Autodesk Inventor part; units mm, degrees
ref_plane "YZ Plane" through (0, 0, 0) normal (1, 0, 0) x (0, 1, 0)
ref_plane "XZ Plane" through (0, 0, 0) normal (0, 1, 0) x (-1, 0, 0)
ref_plane "XY Plane" through (0, 0, 0) normal (0, 0, 1) x (1, 0, 0)
sketch "Sketch1" plane through (0, 0, 0) normal (0, 0, 1) x (1, 0, 0)
  line L0 (-50, -57.5) -> (50, -57.5)
  line L1 (50, -57.5) -> (50, 57.5)
  line L2 (50, 57.5) -> (-50, 57.5)
  line L3 (-50, 57.5) -> (-50, -57.5)
  line L4 (-50, -57.5) -> (50, 57.5) construction
  line L5 (50, -57.5) -> (-50, 57.5) construction
  point P0 (0, 0)
  dimension "d0" = 100
  dimension "d1" = 115
extrude "Plate1" add sketch "Sketch1" along normal blind 3
sketch "Sketch5" plane through (0, 0, 3) normal (0, 0, 1) x (1, 0, 0)
  line L0 (50, -57.5) -> (-50, -57.5) construction
  line L1 (50, 57.5) -> (50, -57.5) construction
  line L2 (-50, 57.5) -> (50, 57.5) construction
  line L3 (-50, -57.5) -> (-50, 57.5) construction
  line L4 (50, 57.5) -> (-50, 57.5) construction
  line L5 (-50, 57.5) -> (50, -57.5) construction
  line L6 (-39.5011, 45.4263) -> (-32.9394, 37.8803) construction
  line L7 (-44.0288, 41.4892) -> (-37.467, 33.9432)
  line L8 (-28.4117, 41.8173) -> (-34.9735, 49.3634)
  arc A0 (-34.9735, 49.3634) -> (-44.0288, 41.4892) centre (-39.5011, 45.4263) ccw
  arc A1 (-37.467, 33.9432) -> (-28.4117, 41.8173) centre (-32.9394, 37.8803) ccw
  point P0 (0, 0)
  point P1 (-36.2202, 41.6533)
  dimension "d22" = 12
  dimension "d23" = 10
  dimension "d24" = 16
extrude "Cut1" cut sketch "Sketch5" against normal blind 3
mirror "Mirror1" about plane through (0, 0, 0) normal (0, 1, 0) of "Cut1"
mirror "Mirror2" about plane through (0, 0, 0) normal (1, 0, 0) of "Cut1", "Mirror1"
fillet "Corner Round1" radius 8 4 edges at (-50, 57.5, 1.5) (50, 57.5, 1.5) (50, -57.5, 1.5) (-50, -57.5, 1.5)
equation "\"d25\" = Thickness"
equation "\"d2\" = Thickness"
equation "\"BendReliefWidth\" = Thickness"
equation "\"BendReliefDepth\" = 0.5 * Thickness"
equation "\"CornerReliefSize\" = 4 * Thickness"
equation "\"MinimumRemnant\" = 2 * Thickness"
equation "\"TransitionRadius\" = BendRadius"
equation "\"JacobiRadiusSize\" = BendRadius"
equation "\"GapSize\" = Thickness"
properties part number "AQUA AISI304 4vv wheel plate 150" material "Stainless Steel"
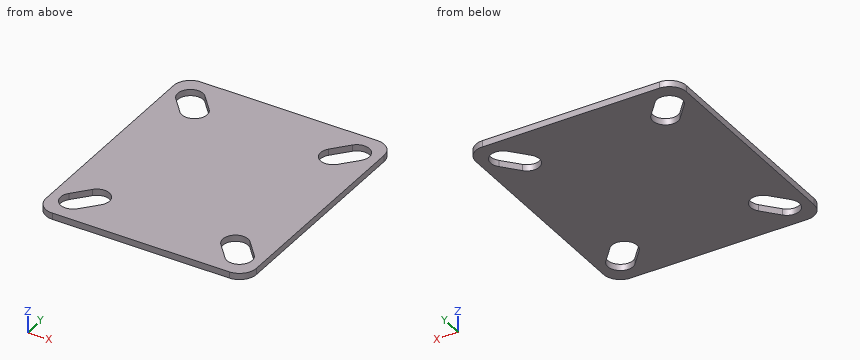
Here's how the part is built. I have some questions about the finished solid (model axes, mm). Coordinates: 2 decimals unless noted, no trailing zeros. Write each loop counter-clockwise with the first axis right and the second up, starting at its lowest first coordinate (ties: lowest second). Pieces come first, ordered by that corner, then holes.
Item 1: I want a section at A-A on z = 1.05. Write out the boundary of the cut face in (x, y).
Item 2: Will this pin go through, and if not, where does the flat tip stop? pin 1 (5 mm diameter, centred on x = 9, y = 16, fed in from -Z).
Item 3: I want a section at C-C on x = -30.5. Write out the boundary of the cut face in (y, z).
Item 4: I want a section at B-B on x = 30. Write out the boundary of the cut face in (y, z), and give its area (3 significant figures).
Item 5: If I drill on line 1 (X direction, y = -39, z = 1.7); line 2 (Y direction, x = 39, z = 0.8); line 3 (Y direction, x = -38, z = 0.95), over which ranges is the centre line in solid material (lowest first)?
Findings below:
1. outline: (-50, -49.5) arc R8 ccw to (-42, -57.5) - (42, -57.5) arc R8 ccw to (50, -49.5) - (50, 49.5) arc R8 ccw to (42, 57.5) - (-42, 57.5) arc R8 ccw to (-50, 49.5) - close; hole (-44.03, -41.49) arc R6 ccw to (-34.97, -49.36) - (-28.41, -41.82) arc R6 ccw to (-37.47, -33.94) - close; hole (-44.03, 41.49) - (-37.47, 33.94) arc R6 ccw to (-28.41, 41.82) - (-34.97, 49.36) arc R6 ccw to start; hole (28.41, -41.82) - (34.97, -49.36) arc R6 ccw to (44.03, -41.49) - (37.47, -33.94) arc R6 ccw to start; hole (28.41, 41.82) arc R6 ccw to (37.47, 33.94) - (44.03, 41.49) arc R6 ccw to (34.97, 49.36) - close
2. pin 1: stops at z = 0
3. outline: (-57.5, 0) - (-44.22, 0) - (-44.22, 3) - (-57.5, 3) - close; (-32.4, 0) - (32.4, 0) - (32.4, 3) - (-32.4, 3) - close; (44.22, 0) - (57.5, 0) - (57.5, 3) - (44.22, 3) - close
4. outline: (-57.5, 0) - (-43.64, 0) - (-43.64, 3) - (-57.5, 3) - close; (-32.65, 0) - (32.65, 0) - (32.65, 3) - (-32.65, 3) - close; (43.64, 0) - (57.5, 0) - (57.5, 3) - (43.64, 3) - close
4. area: 279 mm2
5. line 1: x = -50 to -41.86, -27.04 to 27.04, 41.86 to 50
5. line 2: y = -57.5 to -51.41, -35.71 to 35.71, 51.41 to 57.5
5. line 3: y = -57.5 to -51.24, -34.56 to 34.56, 51.24 to 57.5
